Check sheet for the modelled part. Datum: model origin and axes. Units: mm. Round coordinates to 2 decimals unless told otherwise and drop trailing zeros. Order: outer loops, then holes, each group sorted by start corner. A loop starts at its lowest first (then second) coordinate and runs counter-clockwise, first axis right, second up.
from build123d import *

# Parameters (mm, degrees)
ARRAY_X_COUNT = 3
ARRAY_X_PITCH = 18
ARRAY_Y_COUNT = 3
ARRAY_Y_PITCH = 18
BOX_W         = 56
BOX_H         = 56
BOX_DEPTH     = 10


with BuildPart() as array:
    # Sphere → Sphere (revolve)
    with BuildSketch(Plane.XZ):
        with BuildLine():
            ThreePointArc((0, -8), (8, 0), (0, 8))
            Line((0, 8), (0, -8))
        make_face()
    revolve(axis=Axis((0, 0, 0), (0, 0, 1)))

    # Array X: Array ×3


with BuildPart() as array_1:
    add(array.part)
    with Locations(*[(i * ARRAY_X_PITCH, 0, 0) for i in range(1, ARRAY_X_COUNT)]):
        add(array.part)

    # Array Y: Array ×3


with BuildPart() as array_2:
    add(array_1.part)
    with Locations(*[(0, i * ARRAY_Y_PITCH, 0) for i in range(1, ARRAY_Y_COUNT)]):
        add(array_1.part)


with BuildPart() as array_3:
    # Array placement: moved
    add(array_2.part.moved(Location((10, 10, 10))))


with BuildPart() as porta_bales:
    # Box → Box (new body)
    with BuildSketch(Plane(origin=(-10, -10, -10), x_dir=(1, 0, 0), z_dir=(0, 0, 1))):
        with Locations((28, 28)):
            Rectangle(BOX_W, BOX_H)
    extrude(amount=BOX_DEPTH)

    # Cut: cut Array
    add(array_3.part, mode=Mode.SUBTRACT)


with BuildPart() as porta_bales_1:
    # Cut placement: moved
    add(porta_bales.part.moved(Location((10, 10, 10))))

    # Cut001: cut Array
    add(array_3.part, mode=Mode.SUBTRACT)


solid = porta_bales_1.part
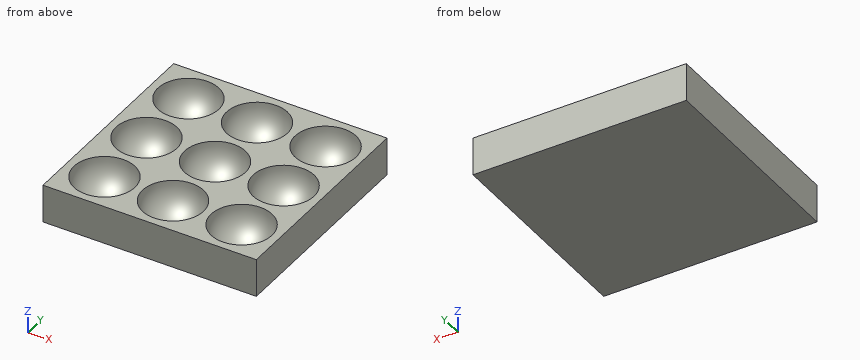
1) Scan lines: line 1 (Y direction, x = 28.5, z = 3); line 2 (Y direction, x = 24, z = 4.5); line 3 (X direction, y = 34, z = 8.25). Record each from-to range of solid material in increasing order.
2) Sectioned sample at A-A on z = 8.75. Count the separate pieces of the cut face and the enclosed holes in it, and give its area (3 significant figures).
3) Sectioned sample at C-C on y = 41.5. Record the cut outline in (x, z), and give its area (3 significant figures).
4) Sectioned sample at B-B on x = 15. Record the cut outline in (y, z) (3 decimals), and give its area (3 significant figures).
Values found:
1. line 1: y = 0 to 6.16, 13.84 to 24.16, 31.84 to 42.16, 49.84 to 56
1. line 2: y = 0 to 5.79, 14.21 to 23.79, 32.21 to 41.79, 50.21 to 56
1. line 3: x = 0 to 5.01, 14.99 to 23.01, 32.99 to 41.01, 50.99 to 56
2. separate pieces: 1
2. enclosed holes: 9
2. area: 1,370 mm2
3. outline: (0, 0) - (56, 0) - (56, 10) - (52.61, 10) arc R6.61 cw to (39.39, 10) - (34.61, 10) arc R6.61 cw to (21.39, 10) - (16.61, 10) arc R6.61 cw to (3.39, 10) - (0, 10) - close
3. area: 354 mm2
4. outline: (0, 0) - (56, 0) - (56, 10) - (52.245, 10) arc R6.245 cw to (39.755, 10) - (34.245, 10) arc R6.245 cw to (21.755, 10) - (16.245, 10) arc R6.245 cw to (3.755, 10) - (0, 10) - close
4. area: 376 mm2
